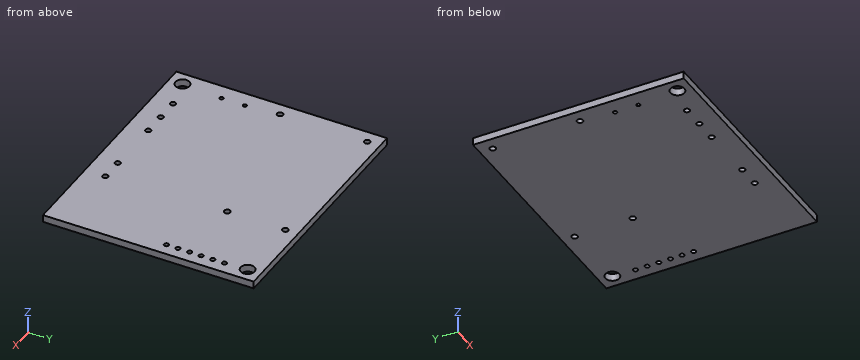
```python
from build123d import *

# Parameters (mm, degrees)
F0_W     = 53.8
F0_H     = 46.05
F0_R     = 1.525
F0_R_2   = 0.6
F0_R_3   = 0.41
F0_R_4   = 0.65
F0_R_5   = 0.5
F1_DEPTH = 1.6


with BuildPart() as f1:
    # F0 (on Top) → F1 (new body)
    with BuildSketch(Plane.XY):
        Rectangle(F0_W, F0_H)
        with Locations((-23.88, -20.035)):
            Circle(F0_R, mode=Mode.SUBTRACT)
        with Locations((-17.29, -18.535)):
            Circle(F0_R_2, mode=Mode.SUBTRACT)
        with Locations((-12.29, -18.535)):
            Circle(F0_R_2, mode=Mode.SUBTRACT)
        with Locations((-7.29, -18.535)):
            Circle(F0_R_2, mode=Mode.SUBTRACT)
        with Locations((-23.34, -11.195)):
            Circle(F0_R_3, mode=Mode.SUBTRACT)
        with Locations((-23.34, -6.115)):
            Circle(F0_R_3, mode=Mode.SUBTRACT)
        with Locations((4.95, -18.585)):
            Circle(F0_R_2, mode=Mode.SUBTRACT)
        with Locations((9.95, -18.585)):
            Circle(F0_R_2, mode=Mode.SUBTRACT)
        with Locations((-24.03, 1.205)):
            Circle(F0_R_4, mode=Mode.SUBTRACT)
        with Locations((-24.03, 20.255)):
            Circle(F0_R_4, mode=Mode.SUBTRACT)
        with Locations((8.99, 7.555)):
            Circle(F0_R_4, mode=Mode.SUBTRACT)
        with Locations((24.2, 2.475)):
            Circle(F0_R_5, mode=Mode.SUBTRACT)
        with Locations((24.2, 5.015)):
            Circle(F0_R_5, mode=Mode.SUBTRACT)
        with Locations((24.2, 7.555)):
            Circle(F0_R_5, mode=Mode.SUBTRACT)
        with Locations((24.2, 10.095)):
            Circle(F0_R_5, mode=Mode.SUBTRACT)
        with Locations((8.99, 20.255)):
            Circle(F0_R_4, mode=Mode.SUBTRACT)
        with Locations((24.2, 12.635)):
            Circle(F0_R_5, mode=Mode.SUBTRACT)
        with Locations((24.2, 15.175)):
            Circle(F0_R_5, mode=Mode.SUBTRACT)
        with Locations((23.91, 20.085)):
            Circle(F0_R, mode=Mode.SUBTRACT)
    extrude(amount=-F1_DEPTH)


solid = f1.part
```
Input: part model. Units: mm. Frame: model coordinates. Coordinates: 2 decimals unless noted, no trailing zeros. Loops run counter-clockwise (first coordinate to the right, second up) from the corner with the lowest first, then second, coordinate; pieces in that order, holes last. Notation, with made-up numbers: M 8.25,52.5 L 26.25,52.5 A8 ccw 26.25,57.5 Z; hole C 21.25,-6 d11. An arc over 180 degrees is marked long. Answer in a Markdown table with one row per item.
1. Section A-A, the plane x = -7.29. Output: boundary loops of the cut face in (y, z) (3 decimals), then the cut area to 3 significant figures.
Response:
| item | result |
|---|---|
| outline | M -23.025,-1.6 L -19.135,-1.6 L -19.135,0 L -23.025,0 Z; M -17.935,-1.6 L 23.025,-1.6 L 23.025,0 L -17.935,0 Z |
| area | 71.8 mm2 |
2. First-contact query: pin 1 (1 mm diameter, centred on x = -7.29, y = -18.535, fed in from -Z). Flat tip, straight axial feed; report the tip coordinate or a pass-through.
Response:
| item | result |
|---|---|
| pin 1 | passes through |
3. Material intervals for line 1 (Y direction, x = -24.03, z = -0.6) (3 decimals); line 2 (Y direction, x = -12.29, z = -1) (3 decimals); line 3 (Y direction, x = 8.5, z = -1.1) (3 decimals), sorted ascending.
Response:
| item | result |
|---|---|
| line 1 | y = -23.025 to -21.553, -18.517 to 0.555, 1.855 to 19.605, 20.905 to 23.025 |
| line 2 | y = -23.025 to -19.135, -17.935 to 23.025 |
| line 3 | y = -23.025 to 7.128, 7.982 to 19.828, 20.682 to 23.025 |
